from build123d import *

# Parameters (mm, degrees)
F0_W     = 40
F0_H     = 40
F1_DEPTH = 140
F2_R     = 5.7
F3_DEPTH = 40
F4_R     = 4
F5_DEPTH = 40
F6_R     = 7
F6_R_2   = 5.7
F7_DEPTH = 12.5
F8_R     = 7
F8_R_2   = 5.7
F9_DEPTH = 12.5


with BuildPart() as f1:
    # F0 (on Front) → F1 (new body)
    with BuildSketch(Plane.XZ):
        Rectangle(F0_W, F0_H)
    extrude(amount=F1_DEPTH)

    # F2 (on face) → F3 (cut)
    with BuildSketch(Plane.XY.offset(20)):
        with Locations((0, -55)):
            Circle(F2_R)
        with Locations((0, -85)):
            Circle(F2_R)
        with Locations((0, -115)):
            Circle(F2_R)
        with Locations((0, -25)):
            Circle(F2_R)
    extrude(amount=-F3_DEPTH, mode=Mode.SUBTRACT)

    # F4 (on face) → F5 (cut)
    with BuildSketch(Plane.YZ.offset(20)):
        with Locations((-130, 10)):
            Circle(F4_R)
        with Locations((-10, -10)):
            Circle(F4_R)
    extrude(amount=-F5_DEPTH, mode=Mode.SUBTRACT)

    # F6 (on face) → F7 (cut)
    with BuildSketch(Plane(origin=(0, 0, -20), x_dir=(1, 0, 0), z_dir=(0, 0, -1))):
        with Locations((0, 115)):
            Circle(F6_R)
        with Locations((0, 115)):
            Circle(F6_R_2, mode=Mode.SUBTRACT)
        with Locations((0, 85)):
            Circle(F6_R)
        with Locations((0, 85)):
            Circle(F6_R_2, mode=Mode.SUBTRACT)
        with Locations((0, 55)):
            Circle(F6_R)
        with Locations((0, 55)):
            Circle(F6_R_2, mode=Mode.SUBTRACT)
        with Locations((0, 25)):
            Circle(F6_R)
        with Locations((0, 25)):
            Circle(F6_R_2, mode=Mode.SUBTRACT)
    extrude(amount=-F7_DEPTH, mode=Mode.SUBTRACT)

    # F8 (on face) → F9 (cut)
    with BuildSketch(Plane.XY.offset(20)):
        with Locations((0, -25)):
            Circle(F8_R)
        with Locations((0, -25)):
            Circle(F8_R_2, mode=Mode.SUBTRACT)
        with Locations((0, -55)):
            Circle(F8_R)
        with Locations((0, -55)):
            Circle(F8_R_2, mode=Mode.SUBTRACT)
        with Locations((0, -85)):
            Circle(F8_R)
        with Locations((0, -85)):
            Circle(F8_R_2, mode=Mode.SUBTRACT)
        with Locations((0, -115)):
            Circle(F8_R)
        with Locations((0, -115)):
            Circle(F8_R_2, mode=Mode.SUBTRACT)
    extrude(amount=-F9_DEPTH, mode=Mode.SUBTRACT)


solid = f1.part
Build history of the part. All positions in model axes, mm. A direction names the side the tool comes from. Coordinates: 2 decimals unless noted, no trailing zeros. Write each loop counter-clockwise with the first axis right and the second up, starting at its lowest first coordinate (ties: lowest second). Pieces come first, ordered by that corner, then holes. Notation, with made-up numbers: (26, 52.25) -> (57, 52.25) arc R16 ccw to (57, 57.25) -> close; hole circle Ø10 at (27.25, -19.5). An arc over 180 degrees is marked (long way). Use CSV: the item, a comma, the result in double quotes. Start each with the question number.
Q1. 3-axis set-ups, long thin cutter, end or side, ignore diameter. For faces 1 (the cylindrical face through (-1.517, -31.834, 13.838)), 2 (the cylindrical face through (-0.74, -19.35, 0.11)), 3 (the cylindrical face through (3.23, -108.79, -13.84)): which of +Z, -Z, +X, -X, +Y, -Y reach the whole face in a straight line?
Q2. Pull direction Y, two halves, no side cores. Call faces 4 (the flat face through (0, -140, 0)), 5 (the cylindrical face through (-1.517, -18.166, -13.838)), 6 (the flat face through (-20, -69, 0)): released by +Y, released by -Y, zero draft, split by the parting line, or undercut.
Q3. Cut at C-C, the plane z = -15.5. List the corners of the cut face in (x, y).
Q4. Cut at D-D, the plane x = 0. State how many separate pieces and enclosed holes the cut face has, then the cut area to 3 significant figures.
Q5. Flat gauge pins, fed straight in: pin 1 Ø7 at (x, y) = (-2.5, -114) entering from +Z; pin 2 Ø12.5 at (x, y) = (0, -25) entering from -Z. Where does each tip first touch, or does it go through?
Q6. Cut at B-B, the plane y = -115. List the corners of the cut face in (x, z).
Q7. Drill centre lines: probe 1 along Y at (x, z) = (0, -2.25); probe 2 along X at (y, z) = (-25, 0); probe 3 along Z at (x, y) = (-7, -130). Where is each one in solid material? Low to high.
Q8. Cut at A-A, the plane z = 10. List the corners of the cut face in (x, y).
Checked values:
1,face 1,"+Z"
1,face 2,"+Z, -Z"
1,face 3,"-Z"
2,face 4,"released by -Y"
2,face 5,"undercut"
2,face 6,"zero draft"
3,outline,"(-20, -140) -> (20, -140) -> (20, 0) -> (-20, 0) -> close; hole circle Ø14 at (0, -115); hole circle Ø14 at (0, -85); hole circle Ø14 at (0, -55); hole circle Ø14 at (0, -25)"
4,separate pieces,"5"
4,enclosed holes,"2"
4,area,"3,420 mm²"
5,pin 1,"stops at z = 7.5"
5,pin 2,"stops at z = -7.5"
6,outline,"(-20, -20) -> (-7, -20) -> (-7, -7.5) -> (-5.7, -7.5) -> (-5.7, 7.5) -> (-7, 7.5) -> (-7, 20) -> (-20, 20) -> close; (5.7, -7.5) -> (7, -7.5) -> (7, -20) -> (20, -20) -> (20, 20) -> (7, 20) -> (7, 7.5) -> (5.7, 7.5) -> close"
7,probe 1,"y = -140 to -120.7, -109.3 to -90.7, -79.3 to -60.7, -49.3 to -30.7, -19.3 to 0"
7,probe 2,"x = -20 to -5.7, 5.7 to 20"
7,probe 3,"z = -20 to 6, 14 to 20"
8,outline,"(-20, -140) -> (20, -140) -> (20, -134) -> (-20, -134) -> close; (-20, -126) -> (20, -126) -> (20, 0) -> (-20, 0) -> close; hole circle Ø14 at (0, -115); hole circle Ø14 at (0, -85); hole circle Ø14 at (0, -55); hole circle Ø14 at (0, -25)"
